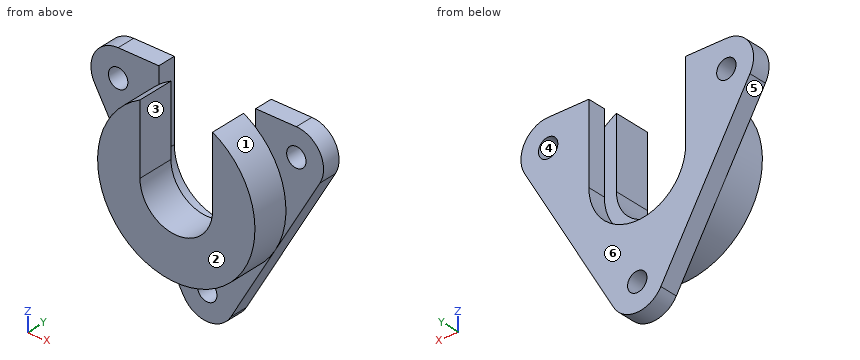
```python
from build123d import *

# Parameters (mm, degrees)
SKETCH_1_R          = 13
SKETCH_1_R_2        = 6
EXTRUDE_1_DEPTH     = 6
SKETCH_2_R          = 8
EXTRUDE_2_DEPTH     = 3
CUT_EXTRUDE_1_DEPTH = 47.127561032
OTHER_START         = -30
OTHER_1_OUTLINE_R   = 1.6
OTHER_1_DEPTH       = 3


# Read off the part's stored shape, not the designer's step: 高级异型孔1
with BuildPart() as part:
    # 草图1 → 凸台-拉伸1 (new body)
    with BuildSketch(Plane(origin=(0, -30, 0), x_dir=(1, 0, 0), z_dir=(0, 1, 0))):
        with Locations(Location((0, 0, 0), (0, 0, 270))):
            Circle(SKETCH_1_R)
        with Locations(Location((0, 0, 0), (0, 0, 270))):
            Circle(SKETCH_1_R_2, mode=Mode.SUBTRACT)
    extrude(amount=-EXTRUDE_1_DEPTH)

    # 草图2 → 凸台-拉伸2 (add)
    with BuildSketch(Plane(origin=(0, -30, 0), x_dir=(1, 0, 0), z_dir=(0, 1, 0))):
        with BuildLine():
            Line((-3.897114317, 19.25), (-18.619546181, -6.25))
            ThreePointArc((-18.619546181, -6.25), (-18.619546181, -10.75), (-14.722431864, -13))
            Line((-14.722431864, -13), (14.722431864, -13))
            ThreePointArc((14.722431864, -13), (18.619546181, -10.75), (18.619546181, -6.25))
            Line((18.619546181, -6.25), (3.897114317, 19.25))
            ThreePointArc((3.897114317, 19.25), (0, 21.5), (-3.897114317, 19.25))
        make_face()
        with Locations(Location((0, 0, 0), (0, 0, 270))):
            Circle(SKETCH_2_R, mode=Mode.SUBTRACT)
    extrude(amount=EXTRUDE_2_DEPTH)

    # 草图3 → 切除-拉伸1 (cut, through all)
    with BuildSketch(Plane.XY):
        Polygon((-8, -27), (-8, -30), (-6, -30), (-6, -36.276321086), (6, -36.276321086), (6, -30), (8, -30), (8, -27), align=None)
    extrude(amount=CUT_EXTRUDE_1_DEPTH, mode=Mode.SUBTRACT)

    # 高级异型孔1 outline → 高级异型孔1 (cut)
    with BuildSketch(Plane(origin=(0, 0, 0), x_dir=(1, 0, 0), z_dir=(0, 1, 0)).offset(OTHER_START)):
        with Locations((-14.722431864, -8.5)):
            Circle(OTHER_1_OUTLINE_R)
        with Locations((14.722431864, -8.5)):
            Circle(OTHER_1_OUTLINE_R)
        with Locations((0, 17)):
            Circle(OTHER_1_OUTLINE_R)
    extrude(amount=OTHER_1_DEPTH, mode=Mode.SUBTRACT)


solid = part.part
```
Part model, mm, in its own coordinate system. Face numbers are marked on the shaded views. A direction names the side the tool comes from. Give positions to 0.01 mm unless a question says otherwise; leave off trailing zeros. Write each loop counter-clockwise with the first axis right and the second up, starting at its lowest first coordinate (ties: lowest second). Pieces come first, ordered by that corner, then holes. Notation, with made-up numbers: M -17,-5 L -13,-5 A36 cw -13,34 Z; hole C 12,45 d5. An arc over 180 degrees is marked long. Use CSV: the item, a comma, the result in double quotes.
Item 1: Pin check, flat tips, straight feed: P1, Ø1.8, axis at y = -31.5, z = 7, coming from the -X side; P2, Ø3, axis at x = 0, z = -17, coming from the +Y side (3 decimals); P3, Ø4, axis at x = -5.5, y = -28.5, coming from the +Z side; P4, Ø1, axis at x = -5.5, y = -29, coming from the -Z side. Stop position of each tip, or through.
Taken from the geometry:
P1,"stops at x = -11.48"
P2,"passes through"
P3,"stops at z = 11.53"
P4,"stops at z = -17.34"
Item 2: Drill centre lines: probe 1 along X at (y, z) = (-28.4, 8.5); probe 2 along X at (y, z) = (-29.5, 9); probe 3 along Y at (x, z) = (-15, 1.5). Where is each one in solid material? Low to high.
Taken from the geometry:
probe 1,"x = -19.22 to -16.32, -13.12 to -8, 8 to 13.12, 16.32 to 19.22"
probe 2,"x = -19.19 to -16.24, -13.2 to -8, 8 to 13.2, 16.24 to 19.19"
probe 3,"y = -30 to -27"
Item 3: Pull direction Z, two halves, no side cores. Call the marked faces 4, 5 and 6: +Z half, -Z half, draft (parallel to the pull), parting line (faces both ways), or undercut.
Taken from the geometry:
face 4,"undercut"
face 5,"-Z half"
face 6,"draft"
Item 4: Slice it at D-D on z = 8.5. Write the cut outline in (x, y), plus the area to 3 significant figures.
Taken from the geometry:
outline,"M -19.22,-30 L -16.32,-30 L -16.32,-27 L -19.22,-27 Z; M -13.12,-30 L -9.84,-30 L -9.84,-36 L -6,-36 L -6,-30 L -8,-30 L -8,-27 L -13.12,-27 Z; M 6,-36 L 9.84,-36 L 9.84,-30 L 13.12,-30 L 13.12,-27 L 8,-27 L 8,-30 L 6,-30 Z; M 16.32,-30 L 19.22,-30 L 19.22,-27 L 16.32,-27 Z"
area,"94.2 mm²"
Item 5: Which spindle directions (+Z, -Z, +X, -X, +Y, -Y) get a long thin tool onto all of the face, cutting with end or side? Do the marked faces 1, 2 and 3. Say none if no direction does.
Taken from the geometry:
face 1,"-Y"
face 2,"+Z, -Z, +X, -X, -Y"
face 3,"+Z, +Y, -Y"
Item 6: Slice it at A-A on x = 0. Write the cut outline in (y, z).
Taken from the geometry:
outline,"M -36,-13 L -30,-13 L -30,-15.4 L -27,-15.4 L -27,-8 L -30,-8 L -30,-6 L -36,-6 Z; M -30,-21.5 L -27,-21.5 L -27,-18.6 L -30,-18.6 Z"
Item 7: Slice it at C-C on z = -17. Write the cut outline in (x, y).
Taken from the geometry:
outline,"M -5.2,-30 L -1.6,-30 L -1.6,-27 L -5.2,-27 Z; M 1.6,-30 L 5.2,-30 L 5.2,-27 L 1.6,-27 Z"
Item 8: Slice it at B-B on y = -28.25. Write the cut outline in (x, z).
Taken from the geometry:
outline,"M -18.62,6.25 L -3.9,-19.25 A4.5 ccw 3.9,-19.25 L 18.62,6.25 A4.5 ccw 14.72,13 L 8,13 L 8,0 A8 cw -8,0 L -8,13 L -14.72,13 A4.5 ccw Z; hole C -14.72,8.5 d3.2; hole C 0,-17 d3.2; hole C 14.72,8.5 d3.2"
